The listing builds one solid part. Answer for the finished solid, in the listing's coordinates (mm). Face numbers are marked on the shaded views. A direction names the side the tool comes from. Give positions to 0.01 mm unless a question says otherwise; leave off trailing zeros. Loops run counter-clockwise (first coordinate to the right, second up) from the corner with the lowest first, then second, coordinate; pieces in that order, holes last.
Item 1: Section C-C, the plane y = 1.5 is taken. Give the vertices of the cut face in (x, z) (3 decimals), and give its area (3 significant figures).
Item 2: A tool of negligible diameter and unlimited length cuts with its end or side. For the marked faces 5 and 6, from which of +Z, -Z, +X, -X, +Y, -Y can it reach the whole face along a straight path? Write none if from no direction.
Item 3: Consider line 1 along X through (y, z) = (27.5, 13.75) (3 decimals); line 2 along Y through (x, z) = (-29, 11.75) (3 decimals); line 3 along X through (y, z) = (-25, 1.75) (3 decimals). Determine where each line is inside the solid, lowest interval first.
Item 4: Each of these flat-tipped pins is pushed along its axis until it touches: pin 1 Ø3 at (x, y) = (36.5, 9) entering from +Z; pin 2 Ø0.8 at (x, y) = (-34.5, -7) entering from +Z; pin 3 Ø3 at (y, z) = (-13.5, 1) entering from -X (3 decimals); pin 4 Ø2 at (y, z) = (28.5, 2) entering from -X (3 decimals). Where does it stop, or does it pass through?
Item 5: Section B-B, the plane x = -28.5 is taken. Give the vertices of the cut face in (y, z) (3 decimals), and give its area (3 significant figures).
Item 6: Section A-A, the plane z = 13.5 is taken. Give the number of separate pieces and of enclosed holes in the cut face, and give its area (3 significant figures).
Item 7: The mould has two halves that part along X. Classify the marked faces 1, 2, 3 and 4: pulls with the +X half, pulls with the -X half, needs draft (parallel to the pull), parting line crosses it, or undercut.
Item 8: Section D-D, the plane x = 21 is taken. Give the vertices of the cut face in (y, z) (3 decimals).
from build123d import *

# Parameters (mm, degrees)
BOSS_EXTRUDE1_DEPTH = 2
SKETCH2_W           = 6.5
SKETCH2_H           = 6.5
SKETCH2_R           = 1.4
BOSS_EXTRUDE2_DEPTH = 18
SKETCH3_W           = 68.5
SKETCH3_H           = 54
CUT_EXTRUDE1_DEPTH  = 1
SNAP_START          = 34.25
SNAP_HOOK1_DEPTH    = 2.753937008
SNAP_START_2        = 7.4782452
SNAP_HOOK1_2_DEPTH  = 3.055920826
SNAP_START_3        = 7.293382709
SNAP_HOOK1_3_DEPTH  = 3.425645808
SNAP_START_4        = 32
SNAP_HOOK1_4_DEPTH  = 7
LPATTERN1_START     = 34.25
LPATTERN1_DEPTH     = 2.753937008
LPATTERN1_START_2   = -17.740925941
LPATTERN1_2_DEPTH   = 3.56278637
LPATTERN1_START_3   = -17.487493169
LPATTERN1_3_DEPTH   = 3.055920826
LPATTERN1_START_4   = 32
LPATTERN1_4_DEPTH   = 7
SNAP_START_5        = -35.757874016
SNAP_HOOK2_DEPTH    = 1.507874016
SNAP_START_6        = -8.712249477
SNAP_HOOK2_2_DEPTH  = 3.415306745
SNAP_START_7        = -8.532556518
SNAP_HOOK2_3_DEPTH  = 3.055920826
SNAP_START_8        = -39
SNAP_HOOK2_4_DEPTH  = 7
BOSS_EXTRUDE3_START = 23
BOSS_EXTRUDE3_DEPTH = 23
SKETCH5_W           = 87.55
SKETCH5_H           = 66.23
CUT_EXTRUDE2_DEPTH  = 2
SKETCH6_W           = 2
SKETCH6_H           = 62.23
BOSS_EXTRUDE4_DEPTH = 1
SKETCH7_W           = 2
SKETCH7_H           = 3
SKETCH7_H_2         = 5
CUT_EXTRUDE3_DEPTH  = 2
SKETCH9_W           = 4
SKETCH9_H           = 2
BOSS_EXTRUDE6_DEPTH = 3


with BuildPart() as part:
    # Sketch1 → Boss-Extrude1 (new body)
    with BuildSketch(Plane.XY):
        with BuildLine():
            Line((-43.275, 35.115), (43.275, 35.115))
            ThreePointArc((43.275, 35.115), (44.689213562, 34.529213562), (45.275, 33.115))
            Line((45.275, 33.115), (45.275, -33.115))
            ThreePointArc((45.275, -33.115), (44.689213562, -34.529213562), (43.275, -35.115))
            Line((43.275, -35.115), (-43.275, -35.115))
            ThreePointArc((-43.275, -35.115), (-44.689213562, -34.529213562), (-45.275, -33.115))
            Line((-45.275, -33.115), (-45.275, 33.115))
            ThreePointArc((-45.275, 33.115), (-44.689213562, 34.529213562), (-43.275, 35.115))
        make_face()
    extrude(amount=-BOSS_EXTRUDE1_DEPTH)

    # Sketch2 → Boss-Extrude2 (add)
    # profile 1 of 4: a face of its own
    with BuildSketch(Plane.XY):
        with Locations((-38.025, -27.865)):
            Rectangle(SKETCH2_W, SKETCH2_H)
        with Locations((-37.465, -27.305)):
            Circle(SKETCH2_R, mode=Mode.SUBTRACT)
    # profile 2 of 4: a face of its own
    with BuildSketch(Plane.XY):
        with Locations((-38.025, 27.865)):
            Rectangle(SKETCH2_W, SKETCH2_H)
        with Locations((-37.465, 27.305)):
            Circle(SKETCH2_R, mode=Mode.SUBTRACT)
    # profile 3 of 4: a face of its own
    with BuildSketch(Plane.XY):
        with Locations((38.025, -27.865)):
            Rectangle(SKETCH2_W, SKETCH2_H)
        with Locations((37.465, -27.305)):
            Circle(SKETCH2_R, mode=Mode.SUBTRACT)
    # profile 4 of 4: a face of its own
    with BuildSketch(Plane.XY):
        with Locations((38.025, 27.865)):
            Rectangle(SKETCH2_W, SKETCH2_H)
        with Locations((37.465, 27.305)):
            Circle(SKETCH2_R, mode=Mode.SUBTRACT)
    extrude(amount=BOSS_EXTRUDE2_DEPTH)

    # Sketch3 → Cut-Extrude1 (cut)
    with BuildSketch(Plane.XY):
        Rectangle(SKETCH3_W, SKETCH3_H)
    extrude(amount=-CUT_EXTRUDE1_DEPTH, mode=Mode.SUBTRACT)

    # Snap Hook1: read off the stored shape, not the designer's step
    # Snap Hook1 outline → Snap Hook1 (add)
    with BuildSketch(Plane.YZ.offset(SNAP_START)):
        Polygon((10.482583566, 4.511638427), (7.52982766, 4.511638427), (7.293382709, 0), (10.719028517, 0), align=None)
    extrude(amount=SNAP_HOOK1_DEPTH)

    # Snap Hook1 2 outline → Snap Hook1 2 (add)
    with BuildSketch(Plane(origin=(0, 0, 0), x_dir=(1, 0, 0), z_dir=(0, 1, 0)).offset(SNAP_START_2)):
        Polygon((34.25, -3.527386458), (33.265748031, -3.527386458), (34.25, -4.511638427), align=None)
        Polygon((38.131846615, 0), (37.003937008, 0), (37.003937008, -4.511638427), align=None)
    extrude(amount=SNAP_HOOK1_2_DEPTH)

    # Snap Hook1 3 outline → Snap Hook1 3 (add)
    with BuildSketch(Plane(origin=(0, 0, 0), x_dir=(1, 0, 0), z_dir=(0, 1, 0)).offset(SNAP_START_3)):
        Polygon((38.131846615, 0), (37.003937008, 0), (37.003937008, -4.511638427), align=None)
    extrude(amount=SNAP_HOOK1_3_DEPTH)

    # Snap Hook1 4 outline → Snap Hook1 4 (cut)
    with BuildSketch(Plane.YZ.offset(SNAP_START_4)):
        Polygon((10.719028517, 0), (10.719028517, 6), (10.404581841, 6), (10.482583566, 4.511638427), align=None)
        Polygon((7.52982766, 4.511638427), (7.607829385, 6), (7.293382709, 6), (7.293382709, 0), align=None)
    extrude(amount=SNAP_HOOK1_4_DEPTH, mode=Mode.SUBTRACT)

    # LPattern1: read off the stored shape, not the designer's step
    # LPattern1 outline → LPattern1 (add)
    with BuildSketch(Plane.YZ.offset(LPATTERN1_START)):
        Polygon((-14.483154803, 5.820037333), (-17.435910709, 5.820037333), (-17.740925941, 0), (-14.178139571, 0), align=None)
    extrude(amount=LPATTERN1_DEPTH)

    # LPattern1 2 outline → LPattern1 2 (add)
    with BuildSketch(Plane(origin=(0, 0, 0), x_dir=(1, 0, 0), z_dir=(0, 1, 0)).offset(LPATTERN1_START_2)):
        Polygon((38.458946341, 0), (37.003937008, 0), (37.003937008, -5.820037333), align=None)
    extrude(amount=LPATTERN1_2_DEPTH)

    # LPattern1 3 outline → LPattern1 3 (add)
    with BuildSketch(Plane(origin=(0, 0, 0), x_dir=(1, 0, 0), z_dir=(0, 1, 0)).offset(LPATTERN1_START_3)):
        Polygon((34.25, -4.835785364), (33.265748031, -4.835785364), (34.25, -5.820037333), align=None)
    extrude(amount=LPATTERN1_3_DEPTH)

    # LPattern1 4 outline → LPattern1 4 (cut)
    with BuildSketch(Plane.YZ.offset(LPATTERN1_START_4)):
        Polygon((-14.178139571, 0), (-14.178139571, 7), (-14.544994026, 7), (-14.483154803, 5.820037333), align=None)
        Polygon((-17.435910709, 5.820037333), (-17.374071486, 7), (-17.740925941, 7), (-17.740925941, 0), align=None)
    extrude(amount=LPATTERN1_4_DEPTH, mode=Mode.SUBTRACT)

    # Snap Hook2: read off the stored shape, not the designer's step
    # Snap Hook2 outline → Snap Hook2 (add)
    with BuildSketch(Plane.YZ.offset(SNAP_START_5)):
        Polygon((-5.528218152, 4.412997898), (-8.480974058, 4.412997898), (-8.712249477, 0), (-5.296942732, 0), align=None)
    extrude(amount=SNAP_HOOK2_DEPTH)

    # Snap Hook2 2 outline → Snap Hook2 2 (add)
    with BuildSketch(Plane(origin=(0, 0, 0), x_dir=(1, 0, 0), z_dir=(0, 1, 0)).offset(SNAP_START_6)):
        Polygon((-35.757874016, -4.412997898), (-35.757874016, 0), (-37.964372965, 0), align=None)
    extrude(amount=SNAP_HOOK2_2_DEPTH)

    # Snap Hook2 3 outline → Snap Hook2 3 (add)
    with BuildSketch(Plane(origin=(0, 0, 0), x_dir=(1, 0, 0), z_dir=(0, 1, 0)).offset(SNAP_START_7)):
        Polygon((-34.25, -3.428745929), (-34.25, -4.412997898), (-33.265748031, -3.428745929), align=None)
    extrude(amount=SNAP_HOOK2_3_DEPTH)

    # Snap Hook2 4 outline → Snap Hook2 4 (cut)
    with BuildSketch(Plane.YZ.offset(SNAP_START_8)):
        Polygon((-8.480974058, 4.412997898), (-8.397802802, 6), (-8.712249477, 6), (-8.712249477, 0), align=None)
        Polygon((-5.611389408, 6), (-5.528218152, 4.412997898), (-5.296942732, 0), (-5.296942732, 6), align=None)
    extrude(amount=SNAP_HOOK2_4_DEPTH, mode=Mode.SUBTRACT)

    # Sketch4 → Boss-Extrude3 (add)
    with BuildSketch(Plane.XY.offset(BOSS_EXTRUDE3_START)):
        with BuildLine():
            Line((-43.275, 35.115), (43.275, 35.115))
            ThreePointArc((43.275, 35.115), (44.689213562, 34.529213562), (45.275, 33.115))
            Line((45.275, 33.115), (45.275, -33.115))
            ThreePointArc((45.275, -33.115), (44.689213562, -34.529213562), (43.275, -35.115))
            Line((43.275, -35.115), (-43.275, -35.115))
            ThreePointArc((-43.275, -35.115), (-44.689213562, -34.529213562), (-45.275, -33.115))
            Line((-45.275, -33.115), (-45.275, -31.115))
            Line((-45.275, -31.115), (-43.275, -31.115))
            Line((-43.275, -31.115), (-43.275, -29.115))
            Line((-43.275, -29.115), (-41.275, -29.115))
            Line((-41.275, -29.115), (-41.275, -31.115))
            Line((-41.275, -31.115), (41.275, -31.115))
            Line((41.275, -31.115), (41.275, 31.115))
            Line((41.275, 31.115), (-41.275, 31.115))
            Line((-41.275, 31.115), (-41.275, 29.115))
            Line((-41.275, 29.115), (-43.275, 29.115))
            Line((-43.275, 29.115), (-43.275, 31.115))
            Line((-43.275, 31.115), (-45.275, 31.115))
            Line((-45.275, 31.115), (-45.275, 33.115))
            ThreePointArc((-45.275, 33.115), (-44.689213562, 34.529213562), (-43.275, 35.115))
        make_face()
    extrude(amount=-BOSS_EXTRUDE3_DEPTH)

    # Sketch5 → Cut-Extrude2 (cut)
    with BuildSketch(Plane.XY.offset(23)):
        with Locations((0, 0.5)):
            Rectangle(SKETCH5_W, SKETCH5_H)
    extrude(amount=-CUT_EXTRUDE2_DEPTH, mode=Mode.SUBTRACT)

    # Sketch6 → Boss-Extrude4 (add)
    with BuildSketch(Plane.XY):
        with Locations((-42.275, 0)):
            Rectangle(SKETCH6_W, SKETCH6_H)
    extrude(amount=BOSS_EXTRUDE4_DEPTH)

    # Sketch7 → Cut-Extrude3 (cut)
    with BuildSketch(Plane.XY):
        with Locations((-44.275, 27.5)):
            Rectangle(SKETCH7_W, SKETCH7_H)
        with Locations((-44.275, -27.5)):
            Rectangle(SKETCH7_W, SKETCH7_H)
        with Locations((-44.275, 0)):
            Rectangle(SKETCH7_W, SKETCH7_H_2)
    extrude(amount=-CUT_EXTRUDE3_DEPTH, mode=Mode.SUBTRACT)

    # Sketch9 → Boss-Extrude6 (add)
    with BuildSketch(Plane.XY):
        with Locations((20.775, 28)):
            Rectangle(SKETCH9_W, SKETCH9_H)
        with Locations((-20.775, 28)):
            Rectangle(SKETCH9_W, SKETCH9_H)
        with Locations((20.775, -28)):
            Rectangle(SKETCH9_W, SKETCH9_H)
        with Locations((-20.775, -28)):
            Rectangle(SKETCH9_W, SKETCH9_H)
    extrude(amount=BOSS_EXTRUDE6_DEPTH)


solid = part.part
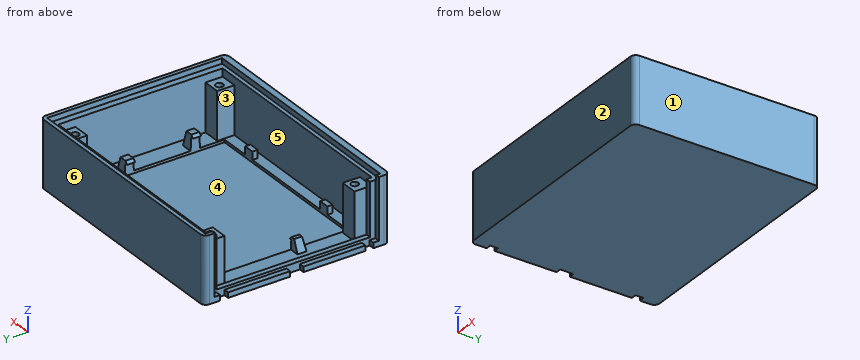
Worked answers:
1. outline: (-43.275, -2) - (45.275, -2) - (45.275, 23) - (43.775, 23) - (43.775, 21) - (41.275, 21) - (41.275, 0) - (34.25, 0) - (34.25, -1) - (-34.25, -1) - (-34.25, 0) - (-41.275, 0) - (-41.275, 1) - (-43.275, 1) - close
1. area: 198 mm2
2. face 5: +Z
2. face 6: +Z, -Z, +X, -X, +Y
3. line 1: x = -41.275 to -38.851, -36.079 to -34.775, 34.775 to 36.079, 38.851 to 45.275
3. line 2: y = -35.115 to -31.115, 31.115 to 35.115
3. line 3: x = -41.275 to -34.775, 34.775 to 45.275
4. pin 1: stops at z = 4.51
4. pin 2: stops at z = 4.41
4. pin 3: stops at x = -45.275
4. pin 4: stops at x = -43.275
5. outline: (-35.115, -2) - (35.115, -2) - (35.115, 23) - (33.615, 23) - (33.615, 21) - (31.115, 21) - (31.115, 0) - (27, 0) - (27, -1) - (-27, -1) - (-27, 0) - (-31.115, 0) - (-31.115, 21) - (-32.615, 21) - (-32.615, 23) - (-35.115, 23) - close
5. area: 262 mm2
6. separate pieces: 1
6. enclosed holes: 4
6. area: 1,120 mm2
7. face 1: pulls with the +X half
7. face 2: needs draft
7. face 3: undercut
7. face 4: undercut
8. outline: (-35.115, -2) - (35.115, -2) - (35.115, 23) - (33.615, 23) - (33.615, 21) - (31.115, 21) - (31.115, 0) - (29, 0) - (29, 3) - (27, 3) - (27, -1) - (-27, -1) - (-27, 3) - (-29, 3) - (-29, 0) - (-31.115, 0) - (-31.115, 21) - (-32.615, 21) - (-32.615, 23) - (-35.115, 23) - close
